Build history of the part. All positions in model axes, mm. A direction names the side the tool comes from. Coordinates: 2 decimals unless noted, no trailing zeros. Loops run counter-clockwise (first coordinate to the right, second up) from the corner with the lowest first, then second, coordinate; pieces in that order, holes last.
Item 1: Cut at A-A (z = 4). List the corners of the cut face in (x, y).
Item 2: 3-axis set-ups, long thin cutter, end or side, ignore diameter. For faces 1 (the face through (-65.031, 5, 4)), 2 (the face through (-103.386, -46, 4)): which of +Z, -Z, +X, -X, +Y, -Y reach the whole face in a straight line?
Item 3: Drill centre lines: line 1 along X through (y, z) = (25.5, 6); line 2 along X through (y, z) = (-6, 3.5); line 3 along Y through (x, z) = (-33, 2.75). Where is each one in solid material? Low to high.
Item 4: Cut at D-D (y = -14). List the corners of the cut face in (x, z).
Item 5: Cut at C-C (x = -84). List the corners of the cut face in (y, z), and give its area (3 significant figures).
Item 6: Mould opens along Y. For faces 3 (the face through (-55, -25, 7.163)), 4 (the face through (-59.403, 25.59, 3.632)), 5 (the face through (-78.34, -48.11, 3.63)), 6 (the face through (-84, -26.582, 4)) say: released by +Y, released by -Y, zero draft, split by the parting line, or undercut.
Item 7: Flat gauge pins, fed straight in: pin 1 (2 mm diameter, centred on x = -75.5, z = 1, fed in from +Y); pin 2 (2 mm diameter, centred on y = -7, z = 3, fed in from -X). Where does each tip first touch, or does it go through?
Item 8: Cut at B-B (x = -56). List the corners of the cut face in (y, z).
Autodesk Inventor part; units mm, degrees
ref_plane "YZ Plane" through (0, 0, 0) normal (1, 0, 0) x (0, 1, 0)
ref_plane "XZ Plane" through (0, 0, 0) normal (0, 1, 0) x (-1, 0, 0)
ref_plane "XY Plane" through (0, 0, 0) normal (0, 0, 1) x (1, 0, 0)
sketch "Sketch1" plane through (0, 0, 0) normal (0, 0, 1) x (1, 0, 0)
  line L0 (-103.3855, 35.2163) -> (-23.0707, 35.2163)
  line L1 (-23.0707, 35.2163) -> (-23.0707, -64.7835)
  line L2 (-23.0707, -64.7835) -> (-103.3855, -64.7835)
  line L3 (-103.3855, -64.7835) -> (-103.3855, 35.2163)
  dimension "d0" = 80.3148
  dimension "d1" = 99.9998
extrude "Extrusion1" add sketch "Sketch1" along normal blind 7.1628
sketch "Sketch2" plane through (0, 0, 7.1628) normal (0, 0, 1) x (1, 0, 0)
  line L0 (-23.0707, 35.2163) -> (-103.3855, 35.2163)
  line L1 (-103.3855, 35.2163) -> (-103.3855, -64.7835)
  line L2 (-103.3855, -64.7835) -> (-23.0707, -64.7835)
  line L3 (-23.0707, -64.7835) -> (-23.0707, 35.2163)
  line L4 (-65.0315, 35.2163) -> (-65.0315, -26.5819)
  line L5 (-103.3855, -26.5819) -> (-65.0315, -26.5819)
  dimension "d4" = 41.9608
  dimension "d5" = 38.2016
extrude "Extrusion2" cut sketch "Sketch2" against normal blind 7.1628 contours L4 L5 L1 L0
sketch "Sketch3" plane through (0, 0, 7.1628) normal (0, 0, 1) x (1, 0, 0)
  line L0 (-23.0707, 35.2163) -> (-65.0315, 35.2163)
  line L1 (-65.0315, -26.5819) -> (-65.0315, -64.7835)
  line L2 (-23.0707, -64.7835) -> (-103.3855, -64.7835)
  circle A0 centre (-84.2085, -45.6827) radius 6.35
  dimension "d8" = 12.7
extrude "Extrusion3" cut sketch "Sketch3" against normal blind 7.1628
sketch "Sketch4" plane through (0, 0, 7.1628) normal (0, 0, 1) x (1, 0, 0)
  line L0 (-65.0315, -26.5819) -> (-65.0315, 35.2163)
  circle A0 centre (-57.0813, 25.4881) radius 2.3241
  circle A1 centre (-31.0209, 25.4881) radius 2.3241
  circle A2 centre (-57.0813, -7.0239) radius 2.3241
  circle A3 centre (-31.0209, -7.0239) radius 2.3241
  dimension "d15" = 4.6482
  dimension "d16" = 4.6482
  dimension "d17" = 4.6482
  dimension "d18" = 4.6482
extrude "Extrusion4" cut sketch "Sketch4" against normal blind 7.1628
properties part number "el torro bracket"
Filled sheet:
1. outline: (-103.39, -64.78) - (-23.07, -64.78) - (-23.07, 35.22) - (-65.03, 35.22) - (-65.03, -26.58) - (-103.39, -26.58) - close; hole circle Ø12.7 at (-84.21, -45.68); hole circle Ø4.65 at (-57.08, -7.02); hole circle Ø4.65 at (-57.08, 25.49); hole circle Ø4.65 at (-31.02, -7.02); hole circle Ø4.65 at (-31.02, 25.49)
2. face 1: +Z, -Z, -X, +Y
2. face 2: +Z, -Z, -X, +Y, -Y
3. line 1: x = -65.03 to -59.41, -54.76 to -33.34, -28.7 to -23.07
3. line 2: x = -65.03 to -59.17, -54.99 to -33.11, -28.93 to -23.07
3. line 3: y = -64.78 to -8.24, -5.81 to 24.27, 26.71 to 35.22
4. outline: (-65.03, 0) - (-23.07, 0) - (-23.07, 7.16) - (-65.03, 7.16) - close
5. outline: (-64.78, 0) - (-52.03, 0) - (-52.03, 7.16) - (-64.78, 7.16) - close; (-39.34, 0) - (-26.58, 0) - (-26.58, 7.16) - (-39.34, 7.16) - close
5. area: 183 mm2
6. face 3: zero draft
6. face 4: undercut
6. face 5: undercut
6. face 6: released by +Y
7. pin 1: stops at y = -26.58
7. pin 2: stops at x = -65.03
8. outline: (-64.78, 0) - (-9.08, 0) - (-9.08, 7.16) - (-64.78, 7.16) - close; (-4.97, 0) - (23.43, 0) - (23.43, 7.16) - (-4.97, 7.16) - close; (27.55, 0) - (35.22, 0) - (35.22, 7.16) - (27.55, 7.16) - close
